Autodesk Inventor part; units mm, degrees
ref_plane "YZ Plane" through (0, 0, 0) normal (1, 0, 0) x (0, 1, 0)
ref_plane "XZ Plane" through (0, 0, 0) normal (0, 1, 0) x (-1, 0, 0)
ref_plane "XY Plane" through (0, 0, 0) normal (0, 0, 1) x (1, 0, 0)
sketch "Sketch1" plane through (0, 0, 0) normal (0, 0, 1) x (1, 0, 0)
  line L0 (3.634, 6.3685) -> (7.3323, 0.0371)
  line L1 (7.3323, 0.0371) -> (3.6983, -6.3314)
  line L2 (3.6983, -6.3314) -> (-3.634, -6.3685)
  line L3 (-3.634, -6.3685) -> (-7.3323, -0.0371)
  line L4 (-7.3323, -0.0371) -> (-3.6983, 6.3314)
  line L5 (-3.6983, 6.3314) -> (3.634, 6.3685)
  point P0 (0, 0)
  point P1 (0, 0)
  dimension "d0" = 12.7
extrude "Extrusion1" add sketch "Sketch1" along normal blind 98.5266
sketch "Sketch2" plane through (0, 0, 98.5266) normal (0, 0, 1) x (1, 0, 0)
  circle A0 centre (0, 0) radius 4.191
  dimension "d3" = 8.382
extrude "Extrusion2" add sketch "Sketch2" along normal blind 2
sketch "Sketch3" plane through (0, 0, 0) normal (0, 0, -1) x (-1, 0, 0)
  circle A0 centre (0, 0) radius 4.191
  dimension "d6" = 8.382
extrude "Extrusion3" add sketch "Sketch3" along normal blind 2
sketch "Sketch4" plane through (0, 0, 100.5266) normal (0, 0, 1) x (1, 0, 0)
  circle A0 centre (0, 0) radius 4.191 construction
  line L0 (7.3323, 0.0371) -> (3.634, 6.3685)
  line L1 (3.634, 6.3685) -> (-3.6983, 6.3314)
  line L2 (-3.6983, 6.3314) -> (-7.3323, -0.0371)
  line L3 (-7.3323, -0.0371) -> (-3.634, -6.3685)
  line L4 (-3.634, -6.3685) -> (3.6983, -6.3314)
  line L5 (3.6983, -6.3314) -> (7.3323, 0.0371)
extrude "Extrusion4" add sketch "Sketch4" along normal blind 6.35
sketch "Sketch5" plane through (0, 0, -2) normal (0, 0, -1) x (-1, 0, 0)
  circle A0 centre (0, 0) radius 4.191 construction
  line L0 (-3.634, 6.3685) -> (-7.3323, 0.0371)
  line L1 (-7.3323, 0.0371) -> (-3.6983, -6.3314)
  line L2 (-3.6983, -6.3314) -> (3.634, -6.3685)
  line L3 (3.634, -6.3685) -> (7.3323, -0.0371)
  line L4 (7.3323, -0.0371) -> (3.6983, 6.3314)
  line L5 (3.6983, 6.3314) -> (-3.634, 6.3685)
extrude "Extrusion5" add sketch "Sketch5" along normal blind 6.35
properties part number "Shafts"
The listing builds one solid part. Answer for the finished solid, in the listing's coordinates (mm). A direction names the side the tool comes from. Give positions to 0.01 mm unless a question says otherwise; leave off trailing zeros. Write each loop counter-clockwise with the first axis right and the second up, starting at its lowest first coordinate (ties: lowest second). Pieces come first, ordered by that corner, then holes. Notation, with made-up numbers: (-32.75, 34.5) - (24.25, 34.5) arc R19 ccw to (24.25, 47.5) - close; hole circle Ø5 at (79, -30.75). An arc over 180 degrees is marked (long way). Use one line per item in the form item = value. Start each with the question number.
1) Find section B-B on z = 31.5. Determine the outline of the cut face in (x, y), plus the area to 3 significant figures.
2) Find section C-C on y = 1. Determine the outline of the cut face in (x, z), plus the area to 3 significant figures.
3) Flat-ended cylindrical pins translate along their axes: pin 1 Ø1 at (x, z) = (-0.5, 18) entering from +Y; pin 2 Ø5 at (y, z) = (-2.5, 75.5) entering from -X; pin 3 Ø2 at (y, z) = (2.5, 37.5) entering from +X. Find the tip coordinate at first contact, or state that the pin passes through.
4) The mould has two halves that part along Z. Classify faces 1 (the face through (-5.51, -3.16, 103.66)), 2 (the face through (0, 0, -8.35)), 3 (the face through (-3.997, -1.259, -0.986)): pulls with the +Z half, pulls with the -Z half, needs draft (parallel to the pull), parting line crosses it, or undercut.
5) Consider line 1 along Z through (x, y) = (0.5, 5.75); line 2 along Y through (x, z) = (1, 30.5); line 3 along Y through (x, z) = (-1, 74.5). Determine where each line is inside the solid, lowest interval first. Write a range as from..to.
6) A tool of negligible diameter and unlimited length cuts with its end or side. For faces 4 (the face through (-2, 4, -2)), 5 (the face through (0, 0, 106.877)), from which of +Z, -Z, +X, -X, +Y, -Y can it reach the whole face along a straight path? Write none if from no direction.
7) Find section D-D on x = 1.25. Determine the outline of the cut face in (y, z), plus the area to 3 significant figures.
8) Find section A-A on x = -6. Determine the outline of the cut face in (y, z).
Geometry results:
q1.outline = (-7.33, -0.04) - (-3.63, -6.37) - (3.7, -6.33) - (7.33, 0.04) - (3.63, 6.37) - (-3.7, 6.33) - close
q1.area = 140 mm2
q2.outline = (-6.74, -8.35) - (6.77, -8.35) - (6.77, -2) - (4.07, -2) - (4.07, 0) - (6.77, 0) - (6.77, 98.53) - (4.07, 98.53) - (4.07, 100.53) - (6.77, 100.53) - (6.77, 106.88) - (-6.74, 106.88) - (-6.74, 100.53) - (-4.07, 100.53) - (-4.07, 98.53) - (-6.74, 98.53) - (-6.74, 0) - (-4.07, 0) - (-4.07, -2) - (-6.74, -2) - close
q2.area = 1,540 mm2
q3.pin_1 = 6.35
q3.pin_2 = -7.33
q3.pin_3 = 6.48
q4.face_1 = needs draft
q4.face_2 = pulls with the -Z half
q4.face_3 = undercut
q5.line_1 = -8.35..-2, 0..98.53, 100.53..106.88
q5.line_2 = -6.35..6.36
q5.line_3 = -6.36..6.35
q6.face_4 = none
q6.face_5 = +Z, +X, -X, +Y, -Y
q7.outline = (-6.34, -8.35) - (6.36, -8.35) - (6.36, -2) - (4, -2) - (4, 0) - (6.36, 0) - (6.36, 98.53) - (4, 98.53) - (4, 100.53) - (6.36, 100.53) - (6.36, 106.88) - (-6.34, 106.88) - (-6.34, 100.53) - (-4, 100.53) - (-4, 98.53) - (-6.34, 98.53) - (-6.34, 0) - (-4, 0) - (-4, -2) - (-6.34, -2) - close
q7.area = 1,440 mm2
q8.outline = (-2.32, -8.35) - (2.3, -8.35) - (2.3, -2) - (-2.32, -2) - close; (-2.32, 0) - (2.3, 0) - (2.3, 98.53) - (-2.32, 98.53) - close; (-2.32, 100.53) - (2.3, 100.53) - (2.3, 106.88) - (-2.32, 106.88) - close
